Source: three-view drawing plus pictorial views. Frame: mm from the lowest corner of the part. A direction names the side the tool comes from. Give positions to 0.01 mm unless a question says otherwise; leave off trailing zeros. Order: outer loops, then holes, each group sorted by start corner. A loop starts at its lowest first (then second) coordinate and runs counter-clockwise, first axis right, second up.
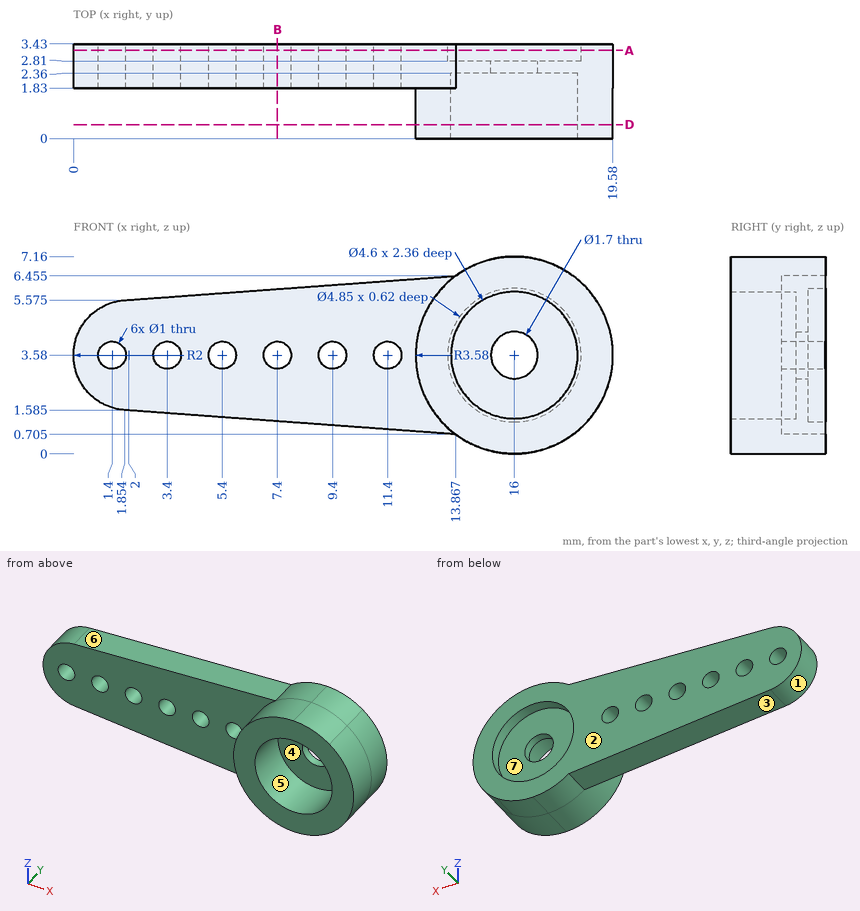
(1) Section D-D, the plane y = 0.5. Return loops of the section in (x, z).
(2) Draft query along Z for the marked faces 1, 2, 3 and 4. Return one class per face: +Z half, -Z half, draft (parallel to the pull), parting line (faces both ways), or undercut.
(3) Pin query (flat end, axial travel): pin 1 Ø1.4 at (x, z) = (16, 3.58) entering from -Y; pin 2 Ø1 at (x, z) = (3.5, 1.5) entering from -Y; pin 3 Ø1.5 at (x, y) = (17.5, 1) entering from +Z. Return the tip coordinate at first contact, or that it passes through.
(4) Section A-A, the plane y = 3.2. Count the separate pieces of the cut face and the enclosed holes in it.
(5) Section B-B, the plane x = 7.4. Return loops of the section in (y, z).
(6) Access query for the marked faces 5, 6 and 7. Directions: +Z, -Z, +X, -X, +Y, -Y. A direction counts if a zero-diameter tool reaches every point of the face in a straight line with its end or side. Return the directions, or none.
(7) Line query: line 1 along Y through (x, z) = (10.5, 5.5); line 2 along Y through (x, z) = (14.5, 4.25); line 3 along Z through (x, y) = (5.4, 2.65) (1 decimal). Output: solid intervals per line, ascending.
Checks:
1. outline: circle Ø7.16 at (16, 3.58); hole circle Ø4.6 at (16, 3.58)
2. face 1: parting line
2. face 2: draft
2. face 3: -Z half
2. face 4: undercut
3. pin 1: passes through
3. pin 2: stops at y = 1.83
3. pin 3: stops at z = 7.08
4. separate pieces: 1
4. enclosed holes: 7
5. outline: (1.83, 1.18) - (3.43, 1.18) - (3.43, 3.08) - (1.83, 3.08) - close; (1.83, 4.08) - (3.43, 4.08) - (3.43, 5.98) - (1.83, 5.98) - close
6. face 5: -Y
6. face 6: +Z, -X, +Y, -Y
6. face 7: +Y
7. line 1: y = 1.83 to 3.43
7. line 2: y = 2.36 to 2.81
7. line 3: z = 1.3 to 3.1, 4.1 to 5.8
